from build123d import *

# Parameters (mm, degrees)
CONNECTOR_PLATE_SKETCH_R      = 85
CONNECTOR_PLATE_EXTRUDE_DEPTH = 20
CONNECTOR_PLATE_SHELL_T       = -10
TRIANGLE_START                = 17
TRIANGLE_SKETCH_R             = 15
TRIANGLE_EXTRUDE_1_DEPTH      = 20
TRIANGLE_START_2              = -37
TRIANGLE_SKETCH_3_R           = 15
TRIANGLE_EXTRUDE_2_DEPTH      = 20
TRIANGLE_FILLET_R             = 30


with BuildPart() as part:
    # Connector Plate Sketch → Connector Plate Extrude (new body)
    with BuildSketch(Plane(origin=(0, 0, 0), x_dir=(1, 0, 0), z_dir=(0, 1, 0))):
        with Locations(Location((0, 0, 0), (0, 0, 270))):
            Circle(CONNECTOR_PLATE_SKETCH_R)
    extrude(amount=CONNECTOR_PLATE_EXTRUDE_DEPTH)

    # Connector Plate Shell
    connector_plate_shell_openings = [part.faces().sort_by_distance(p)[0] for p in [
        (0, 20, 0),
    ]]
    offset(amount=CONNECTOR_PLATE_SHELL_T, openings=connector_plate_shell_openings, kind=Kind.INTERSECTION)

    # Triangle Sketch → Triangle Extrude 1 (add)
    with BuildSketch(Plane(origin=(0, 0, 0), x_dir=(0, 0, -1), z_dir=(1, 0, 0)).offset(TRIANGLE_START)):
        Polygon((65, -100), (-65, 0), (65, 0), align=None)
        with Locations((35, -39.074108923)):
            Circle(TRIANGLE_SKETCH_R, mode=Mode.SUBTRACT)
    extrude(amount=TRIANGLE_EXTRUDE_1_DEPTH)

    # Triangle Sketch_3 → Triangle Extrude 2 (add)
    with BuildSketch(Plane(origin=(0, 0, 0), x_dir=(0, 0, -1), z_dir=(1, 0, 0)).offset(TRIANGLE_START_2)):
        Polygon((65, -100), (-65, 0), (65, 0), align=None)
        with Locations((35, -39.074108923)):
            Circle(TRIANGLE_SKETCH_3_R, mode=Mode.SUBTRACT)
    extrude(amount=TRIANGLE_EXTRUDE_2_DEPTH)

    # Triangle Fillet
    triangle_fillet_edges = [part.edges().sort_by_distance(p)[0] for p in [
        (27, -100, -65),
        (-27, -100, -65),
    ]]
    fillet(triangle_fillet_edges, radius=TRIANGLE_FILLET_R)


solid = part.part
The model under review builds one solid part; all positions refer to its coordinate system, in mm. A direction names the side the tool comes from. Give positions to 0.01 mm unless a question says otherwise; leave off trailing zeros. Order: outer loops, then holes, each group sorted by start corner. A loop starts at its lowest first (then second) coordinate and runs counter-clockwise, first axis right, second up. Notation, with made-up numbers: (15.5, 18.25) -> (31.5, 18.25) arc R13 cw to (31.5, 38.25) -> close; hole circle Ø5 at (38, -24.5). An arc over 180 degrees is marked (long way). Write item = value, one per line. Start each with the question number.
(1) Take a section at A-A (y = -10). Write out the cut boundary in (x, z), plus the area to 3 significant figures.
(2) Take a section at B-B (x = -25). Write out the cut boundary in (y, z).
(3) For pin 1 Ø1 at (x, z) = (-17, 23.5) entering from +Y; pin 2 Ø2 at (y, z) = (10, 36.5) entering from -X; pin 3 Ø20.5 at (y, z) = (-34.5, -19) entering from -X; pin 4 Ø24 at (y, z) = (-39.07, -35) entering from +X, all flat-tipped, find the tip position at first contact; note any pin that passes through.
(4) For L1, parallel to X at y = -7, z = 47; L2, parallel to Y at x = 21.5, z = -35; L3, parallel to X at y = 13.75, z = 0, list the stretches that pass through material, from the lowest coordinate up. Write a range as from..to.
(5) Take a section at D-D (y = -36). Write out the cut boundary in (x, z).
(6) Take a section at C-C (z = 0). Write out the cut boundary in (x, y).
(7) Tool access review of faces 5 (the cylindrical face through (-45.636, 14.93, -59.517)), 6 (the flat face through (-37, -26, -15)), 7 (the flat face through (17, -26, -15)): name each direction out of +Z, -Z, +X, -X, +Y, -Y from which nothing blocks a thin tool from reaching the whole face with its end or side.
(8) Draft analysis for pull direction Z (two halves, no side actions). For faces 1 (the flat face through (26.86, -31.87, 23.57)), 2 (the flat face through (-27, -19, -65)), 3 (the cylindrical face through (-26.86, -66.19, -47.83)), 4 (the flat face through (1, 10, -1)), state which applies: +Z half, -Z half, draft (parallel to the pull), parting line (faces both ways), or undercut.
Returned:
q1.outline = (-37, -65) -> (-17, -65) -> (-17, 52) -> (-37, 52) -> close; (17, -65) -> (37, -65) -> (37, 52) -> (17, 52) -> close
q1.area = 4,680 mm²
q2.outline = (-62.85, -16.71) arc R30 ccw to (-39.07, -65) -> (0, -65) -> (0, -81.24) -> (20, -81.24) -> (20, -70.71) -> (10, -70.71) -> (10, 70.71) -> (20, 70.71) -> (20, 81.24) -> (0, 81.24) -> (0, 65) -> close; hole circle Ø30 at (-39.07, -35)
q3.pin_1 = 10
q3.pin_2 = -77.23
q3.pin_3 = -37
q3.pin_4 = through
q4.L1 = -37..-17, 17..37
q4.L2 = -69.07..-54.07, -24.07..10
q4.L3 = -85..-75, 75..85
q5.outline = (-37, -65) -> (-17, -65) -> (-17, -49.68) -> (-37, -49.68) -> close; (-37, -20.32) -> (-17, -20.32) -> (-17, 18.2) -> (-37, 18.2) -> close; (17, -65) -> (37, -65) -> (37, -49.68) -> (17, -49.68) -> close; (17, -20.32) -> (37, -20.32) -> (37, 18.2) -> (17, 18.2) -> close
q6.outline = (-85, 0) -> (-37, 0) -> (-37, -50) -> (-17, -50) -> (-17, 0) -> (17, 0) -> (17, -50) -> (37, -50) -> (37, 0) -> (85, 0) -> (85, 20) -> (75, 20) -> (75, 10) -> (-75, 10) -> (-75, 20) -> (-85, 20) -> close
q7.face_5 = +Y
q7.face_6 = +Z, -Z, -X, -Y
q7.face_7 = +Z, -Z, -Y
q8.face_1 = +Z half
q8.face_2 = -Z half
q8.face_3 = parting line
q8.face_4 = undercut
